from build123d import *

# Parameters (mm, degrees)
F0_R     = 0.9
F0_R_2   = 1.125
F1_DEPTH = 1
F2_ANGLE = 90
F3_ANGLE = -90


with BuildPart() as f1:
    # F0 (on Right) → F1 (new body)
    with BuildSketch(Plane.YZ):
        with BuildLine():
            ThreePointArc((0, 3), (0.87868, 0.87868), (3, 0))
            Line((3, 0), (98, 0))
            ThreePointArc((98, 0), (100.12132, 0.87868), (101, 3))
            Line((101, 3), (101, 23.63))
            ThreePointArc((101, 23.63), (100.12132, 25.75132), (98, 26.63))
            Line((98, 26.63), (86.95, 26.63))
            Line((86.95, 26.63), (86.95, 10.52))
            Line((86.95, 10.52), (82.55, 10.52))
            Line((82.55, 10.52), (82.55, 26.63))
            Line((82.55, 26.63), (79.4, 26.63))
            Line((79.4, 26.63), (79.4, 9.52))
            Line((79.4, 9.52), (75, 9.52))
            Line((75, 9.52), (75, 26.63))
            Line((75, 26.63), (71.85, 26.63))
            Line((71.85, 26.63), (71.85, 7.56))
            Line((71.85, 7.56), (67.45, 7.56))
            Line((67.45, 7.56), (67.45, 26.63))
            Line((67.45, 26.63), (64.3, 26.63))
            Line((64.3, 26.63), (64.3, 6.5))
            Line((64.3, 6.5), (59.9, 6.5))
            Line((59.9, 6.5), (59.9, 26.63))
            Line((59.9, 26.63), (56.75, 26.63))
            Line((56.75, 26.63), (56.75, 5.63))
            Line((56.75, 5.63), (52.35, 5.63))
            Line((52.35, 5.63), (52.35, 26.63))
            Line((52.35, 26.63), (49.2, 26.63))
            Line((49.2, 26.63), (49.2, 5.39))
            Line((49.2, 5.39), (44.8, 5.39))
            Line((44.8, 5.39), (44.8, 26.63))
            Line((44.8, 26.63), (41.65, 26.63))
            Line((41.65, 26.63), (41.65, 4.63))
            Line((41.65, 4.63), (37.25, 4.63))
            Line((37.25, 4.63), (37.25, 26.63))
            Line((37.25, 26.63), (34.1, 26.63))
            Line((34.1, 26.63), (34.1, 4.63))
            Line((34.1, 4.63), (29.7, 4.63))
            Line((29.7, 4.63), (29.7, 26.63))
            Line((29.7, 26.63), (26.55, 26.63))
            Line((26.55, 26.63), (26.55, 3.63))
            Line((26.55, 3.63), (22.15, 3.63))
            Line((22.15, 3.63), (22.15, 26.63))
            Line((22.15, 26.63), (19, 26.63))
            Line((19, 26.63), (19, 3.13))
            Line((19, 3.13), (14.6, 3.13))
            Line((14.6, 3.13), (14.6, 26.63))
            Line((14.6, 26.63), (3, 26.63))
            ThreePointArc((3, 26.63), (0.87868, 25.75132), (0, 23.63))
            Line((0, 23.63), (0, 3))
        make_face()
        with Locations((50.800736, 6.63)):
            Circle(F0_R, mode=Mode.SUBTRACT)
        with Locations((5, 15.63)):
            Circle(F0_R_2, mode=Mode.SUBTRACT)
        with Locations((96, 15.63)):
            Circle(F0_R_2, mode=Mode.SUBTRACT)
        with Locations((50.7, 22.63)):
            Circle(F0_R, mode=Mode.SUBTRACT)
    extrude(amount=F1_DEPTH)


with BuildPart() as f1_1:
    # F2: moved
    add(f1.part.rotate(Axis((1, 50.5, 0), (0, 1, 0)), F2_ANGLE))


with BuildPart() as f1_2:
    # F3: moved
    add(f1_1.part.rotate(Axis((4, 3, 1), (0, 0, 1)), F3_ANGLE))


with BuildPart() as f1_3:
    # F4: moved
    add(f1_2.part.moved(Location((0, -6, 0))))


with BuildPart() as f1_4:
    # F5: moved
    add(f1_3.part.moved(Location((-1, 0, 0))))


solid = f1_4.part
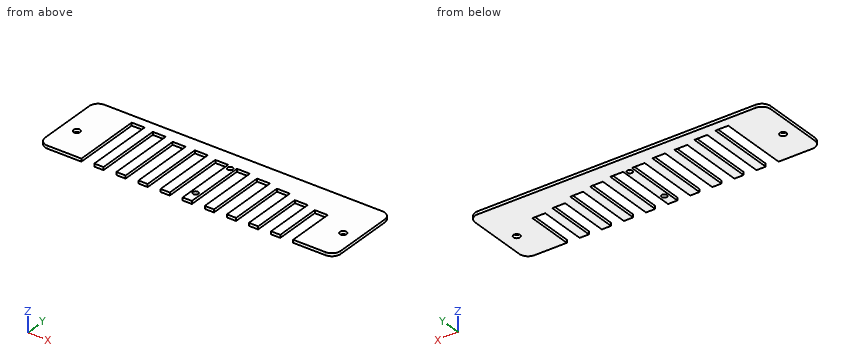
Design review of the part built by this model. Coordinates are the model's own, in mm. Round coordinates to 2 decimals unless told otherwise and drop trailing zeros. Write each loop counter-clockwise with the first axis right and the second up, starting at its lowest first coordinate (ties: lowest second). Pieces come first, ordered by that corner, then holes. Notation, with made-up numbers: (87.25, 70) - (99.25, 70) arc R5 ccw to (99.25, 78) - close; hole circle Ø10 at (77, 57). An arc over 180 degrees is marked (long way). Use a Markdown table: item, result. Add a question column.
1. Clearance check with flat-ended pins moving along their axes: pin 1 (0.5 mm diameter, centred on x = 61.5, z = 0.5, fed in from -Y); pin 2 (1 mm diameter, centred on x = 76.5, y = -19.5, fed in from -Z). State where each tip first meets the part, or that it passes through.
2. Wall thickness on probe 1 along Y at (x, z) = (50.7, 0.4); probe 2 along Y at (x, z) = (5, 0.4) (3 decimals); probe 3 along Y at (x, z) = (23, 0.4): over which ranges is each line inside the solid? List them lowest first.
3. We need section B-B (y = -15.63). Count the separate pieces of the cut face and the enclosed holes in it, then the cut area to 3 significant figures.
4. We need section A-A (x = 96). State the section outline as (y, z) points (3 decimals).
Output:
| question | item | result |
|---|---|---|
| 1 | pin 1 | stops at y = -6.5 |
| 1 | pin 2 | passes through |
| 2 | probe 1 | y = -26.63 to -23.53, -21.73 to -7.52, -5.74 to 0 |
| 2 | probe 2 | y = -26.63 to -16.755, -14.505 to 0 |
| 2 | probe 3 | y = -3.63 to 0 |
| 3 | separate pieces | 13 |
| 3 | enclosed holes | 0 |
| 3 | area | 52.5 mm2 |
| 4 | outline | (-26.63, 0) - (-16.755, 0) - (-16.755, 1) - (-26.63, 1) - close; (-14.505, 0) - (0, 0) - (0, 1) - (-14.505, 1) - close |
